Design review of the part built by this model. Coordinates are the model's own, in mm. Coordinates: 2 decimals unless noted, no trailing zeros. Write each loop counter-clockwise with the first axis right and the second up, starting at its lowest first coordinate (ties: lowest second). Pieces come first, ordered by that corner, then holes. Notation, with made-up numbers: (11, 89) - (52, 89) arc R16 ccw to (52, 113) - close; hole circle Ø2 at (70, 15). An arc over 180 degrees is marked (long way). One line per item, written item: value.
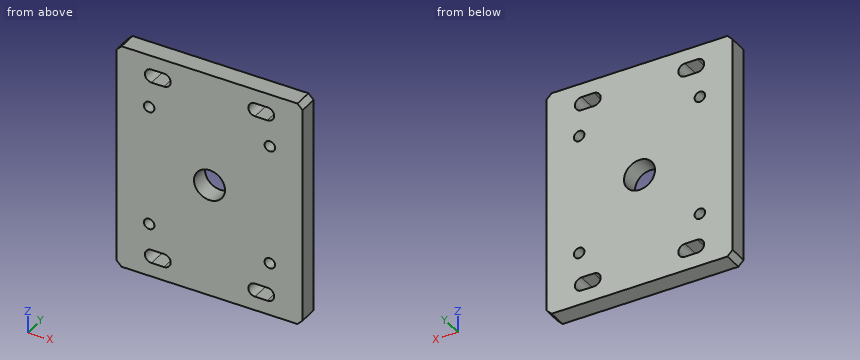
from build123d import *

# Parameters (mm, degrees)
SKETCH_1_W          = 220
SKETCH_1_H          = 18
EXTRUDE_1_DEPTH     = 90
CUT_EXTRUDE_1_REACH = 145.262
SKETCH_2_R          = 15
CHAMFER_1_SIZE      = 5
CUT_EXTRUDE_3_REACH = 145.262
HOLE_WIZARD_M12_1_D = 10.2


with BuildPart() as part:
    # 草圖1 → 伸長1 (new, symmetric)
    with BuildSketch(Plane(origin=(0, 0, 0), x_dir=(0, 0, -1), z_dir=(1, 0, 0))):
        with Locations((0, 9)):
            Rectangle(SKETCH_1_W, SKETCH_1_H)
    extrude(amount=EXTRUDE_1_DEPTH, both=True)

    # 草圖2 → 除料-伸長1 (cut, up to next)
    with BuildSketch(Plane.XZ, mode=Mode.PRIVATE) as cut_extrude_1_sk1:
        with Locations(Location((0, 0, 0), (0, 0, 270))):
            Circle(SKETCH_2_R)
    cut_extrude_1_tool1 = extrude(cut_extrude_1_sk1.sketch, amount=-CUT_EXTRUDE_1_REACH, mode=Mode.PRIVATE) & part.part
    add(cut_extrude_1_tool1.solids().sort_by_distance((0, 0, 0))[0], mode=Mode.SUBTRACT)

    # 導角1
    chamfer_1_edges = [part.edges().sort_by_distance(p)[0] for p in [
        (90, 9, 110),
        (90, 9, -110),
        (-90, 9, 110),
        (-90, 9, -110),
    ]]
    chamfer(chamfer_1_edges, length=CHAMFER_1_SIZE)

    # 草圖4 → 除料-伸長3 (cut, up to next)
    with BuildSketch(Plane.XZ, mode=Mode.PRIVATE) as cut_extrude_3_sk1:
        with BuildLine():
            Line((44, 83.5), (56, 83.5))
            ThreePointArc((56, 83.5), (62.5, 90), (56, 96.5))
            Line((56, 96.5), (44, 96.5))
            ThreePointArc((44, 96.5), (37.5, 90), (44, 83.5))
        make_face()
    cut_extrude_3_tool1 = extrude(cut_extrude_3_sk1.sketch, amount=-CUT_EXTRUDE_3_REACH, mode=Mode.PRIVATE) & part.part
    # 草圖4 → 除料-伸長3 (cut, up to next)
    with BuildSketch(Plane.XZ, mode=Mode.PRIVATE) as cut_extrude_3_sk2:
        with BuildLine():
            Line((-56, 83.5), (-44, 83.5))
            ThreePointArc((-44, 83.5), (-37.5, 90), (-44, 96.5))
            Line((-44, 96.5), (-56, 96.5))
            ThreePointArc((-56, 96.5), (-62.5, 90), (-56, 83.5))
        make_face()
    cut_extrude_3_tool2 = extrude(cut_extrude_3_sk2.sketch, amount=-CUT_EXTRUDE_3_REACH, mode=Mode.PRIVATE) & part.part
    # 草圖4 → 除料-伸長3 (cut, up to next)
    with BuildSketch(Plane.XZ, mode=Mode.PRIVATE) as cut_extrude_3_sk3:
        with BuildLine():
            Line((-56, -96.5), (-44, -96.5))
            ThreePointArc((-44, -96.5), (-37.5, -90), (-44, -83.5))
            Line((-44, -83.5), (-56, -83.5))
            ThreePointArc((-56, -83.5), (-62.5, -90), (-56, -96.5))
        make_face()
    cut_extrude_3_tool3 = extrude(cut_extrude_3_sk3.sketch, amount=-CUT_EXTRUDE_3_REACH, mode=Mode.PRIVATE) & part.part
    # 草圖4 → 除料-伸長3 (cut, up to next)
    with BuildSketch(Plane.XZ, mode=Mode.PRIVATE) as cut_extrude_3_sk4:
        with BuildLine():
            Line((44, -96.5), (56, -96.5))
            ThreePointArc((56, -96.5), (62.5, -90), (56, -83.5))
            Line((56, -83.5), (44, -83.5))
            ThreePointArc((44, -83.5), (37.5, -90), (44, -96.5))
        make_face()
    cut_extrude_3_tool4 = extrude(cut_extrude_3_sk4.sketch, amount=-CUT_EXTRUDE_3_REACH, mode=Mode.PRIVATE) & part.part
    add(cut_extrude_3_tool1.solids().sort_by_distance((50, 0, 90))[0], mode=Mode.SUBTRACT)
    add(cut_extrude_3_tool2.solids().sort_by_distance((-50, 0, 90))[0], mode=Mode.SUBTRACT)
    add(cut_extrude_3_tool3.solids().sort_by_distance((-50, 0, -90))[0], mode=Mode.SUBTRACT)
    add(cut_extrude_3_tool4.solids().sort_by_distance((50, 0, -90))[0], mode=Mode.SUBTRACT)

    # M12 螺紋孔1 (through all)
    with Locations(Plane(origin=(0, 18, 0), x_dir=(-1, 0, 0), z_dir=(0, 1, 0))):
        with Locations((58.336309448, 58.336309448), (58.336309448, -58.336309448), (-58.336309448, -58.336309448), (-58.336309448, 58.336309448)):
            Hole(HOLE_WIZARD_M12_1_D / 2)


solid = part.part
1. Consider section D-D, the plane y = 11.5. Give the number of separate pieces and of enclosed holes in the cut face, then the cut area to 3 significant figures.
Answer block:
separate pieces: 1
enclosed holes: 9
area: 37,400 mm^2
2. Consider section B-B, the plane z = 0. Write out the cut boundary in (x, y), then the cut area to 3 significant figures.
Answer block:
outline: (-90, 0) - (-15, 0) - (-15, 18) - (-90, 18) - close; (15, 0) - (90, 0) - (90, 18) - (15, 18) - close
area: 2,700 mm^2
3. Consider section C-C, the plane z = 90. Write out the cut boundary in (x, y).
Answer block:
outline: (-90, 0) - (-62.5, 0) - (-62.5, 18) - (-90, 18) - close; (-37.5, 0) - (37.5, 0) - (37.5, 18) - (-37.5, 18) - close; (62.5, 0) - (90, 0) - (90, 18) - (62.5, 18) - close
4. Wall thickness on line 1 along Z through (x, y) = (-51.5, 11.75); line 2 along X through (y, z) = (5, 0); line 3 along Z through (x, y) = (-1, 6.5): over which ranges is each line inside the solid? List them lowest first.
Answer block:
line 1: z = -110 to -96.5, -83.5 to 83.5, 96.5 to 110
line 2: x = -90 to -15, 15 to 90
line 3: z = -110 to -14.97, 14.97 to 110
5. Consider section A-A, the plane x = 0. Write out the cut boundary in (y, z).
Answer block:
outline: (0, -110) - (18, -110) - (18, -15) - (0, -15) - close; (0, 15) - (18, 15) - (18, 110) - (0, 110) - close
